Build history of the part. All positions in model axes, mm. A direction names the side the tool comes from. Give positions to 0.01 mm unless a question says otherwise; leave off trailing zeros. Order: outer loops, then holes, each group sorted by start corner. A loop starts at its lowest first (then second) coordinate and runs counter-clockwise, first axis right, second up. Notation, with made-up numbers: (48, 4) -> (104, 4) arc R24 cw to (104, 23) -> close; hole circle Ø10 at (-30.5, 24.25). An arc over 180 degrees is marked (long way). Write item = value, one per line. Start each with the question number.
from build123d import *

# Parameters (mm, degrees)
SKETCH_1_W                = 266.4
SKETCH_1_H                = 50
EXTRUDE_1_DEPTH           = 22
SKETCH_2_W                = 25.2
SKETCH_2_H                = 16
CUT_EXTRUDE_1_DEPTH       = 144.966107122
SKETCH_5_W                = 130
SKETCH_5_H                = 43
CUT_EXTRUDE_4_DEPTH       = 10
CUT_EXTRUDE_2_DEPTH       = 138.299817917
EXTRUDE_2_DEPTH           = 22
CUT_EXTRUDE_5_DEPTH       = 250
HOLE_WIZARD_1_D           = 11
HOLE_WIZARD_1_DEPTH       = 100
HOLE_WIZARD_1_CBORE_D     = 17.5
HOLE_WIZARD_1_CBORE_DEPTH = 11
SKETCH_10_R               = 10
CUT_EXTRUDE_6_DEPTH       = 2
M6X1_0_1_AT_2_COUNT       = 2
M6X1_0_1_AT_2_PITCH       = 35
FILLET_1_R                = 3


with BuildPart() as part:
    # 草图1 → 凸台-拉伸1 (new body)
    with BuildSketch(Plane.XY):
        Rectangle(SKETCH_1_W, SKETCH_1_H)
    extrude(amount=-EXTRUDE_1_DEPTH)

    # 草图2 → 切除-拉伸1 (cut, through all)
    with BuildSketch(Plane(origin=(0, 25, 0), x_dir=(1, 0, 0), z_dir=(0, 1, 0))):
        with Locations((-120.6, 14)):
            Rectangle(SKETCH_2_W, SKETCH_2_H)
        with Locations((120.6, 14)):
            Rectangle(SKETCH_2_W, SKETCH_2_H)
    extrude(amount=-CUT_EXTRUDE_1_DEPTH, mode=Mode.SUBTRACT)

    # 草图5 → 切除-拉伸4 (cut)
    with BuildSketch(Plane(origin=(0, 0, -22), x_dir=(-1, 0, 0), z_dir=(0, 0, -1))):
        with Locations((0, 3.5)):
            Rectangle(SKETCH_5_W, SKETCH_5_H)
    extrude(amount=-CUT_EXTRUDE_4_DEPTH, mode=Mode.SUBTRACT)

    # 草图3 → 切除-拉伸2 (cut, through all)
    with BuildSketch(Plane.XY):
        with BuildLine():
            Line((-42, 25), (-42, -5.726706901))
            ThreePointArc((-42, -5.726706901), (0, -18), (42, -5.726706901))
            Line((42, -5.726706901), (42, 25))
            Line((42, 25), (-42, 25))
        make_face()
    extrude(amount=-CUT_EXTRUDE_2_DEPTH, mode=Mode.SUBTRACT)

    # 草图6 → 凸台-拉伸2 (add)
    with BuildSketch(Plane.XY):
        with BuildLine():
            Line((-52.5, -25), (52.5, -25))
            ThreePointArc((52.5, -25), (0, -39.889777347), (-52.5, -25))
        make_face()
    extrude(amount=-EXTRUDE_2_DEPTH)

    # 草图7 → 切除-拉伸5 (cut, symmetric)
    with BuildSketch(Plane(origin=(0, 0, 0), x_dir=(0, 0, -1), z_dir=(1, 0, 0))):
        Polygon((22, -39.889777347), (22, -26.889777347), (9, -39.889777347), align=None)
        Polygon((0, -39.889777347), (2.7, -39.889777347), (0, -28.889777347), align=None)
    extrude(amount=CUT_EXTRUDE_5_DEPTH, both=True, mode=Mode.SUBTRACT)

    # 孔1
    with Locations(Plane.XY):
        with Locations((80, 0), (-80, 0)):
            CounterBoreHole(HOLE_WIZARD_1_D / 2, HOLE_WIZARD_1_CBORE_D / 2, HOLE_WIZARD_1_CBORE_DEPTH, depth=HOLE_WIZARD_1_DEPTH)

    # 草图10 → 切除-拉伸6 (cut)
    with BuildSketch(Plane(origin=(0, 0, -22), x_dir=(-1, 0, 0), z_dir=(0, 0, -1))):
        with Locations((80, 0)):
            Circle(SKETCH_10_R)
        with Locations((-80, 0)):
            Circle(SKETCH_10_R)
    extrude(amount=-CUT_EXTRUDE_6_DEPTH, mode=Mode.SUBTRACT)

    # 草图11 → M6x1.0 螺纹孔1 (revolve, cut)
    with BuildSketch(Plane(origin=(-108, -17.5, -13.5), x_dir=(0, 0, 1), z_dir=(0, 1, 0))):
        Polygon((0, 0), (0, 16.502151548), (2.5, 15), (2.5, 0), align=None)
    m6x1_0_1 = revolve(axis=Axis((-114.35, -17.5, -13.5), (1, 0, 0)), mode=Mode.SUBTRACT)

    # M6x1.0 螺纹孔1 at 2: M6x1.0 螺纹孔1 ×2
    with Locations(*[(0, i * M6X1_0_1_AT_2_PITCH, 0) for i in range(1, M6X1_0_1_AT_2_COUNT)]):
        add(m6x1_0_1, mode=Mode.SUBTRACT)

    # 镜向1: M6x1.0 螺纹孔1 across plane
    add(m6x1_0_1.mirror(Plane(origin=(0, 0, 0), x_dir=(0, 0, 1), z_dir=(1, 0, 0))), mode=Mode.SUBTRACT)

    # 镜向1 copy 1 sketch → 镜向1 copy 1 (revolve, cut)
    with BuildSketch(Plane(origin=(108, 17.5, -13.5), x_dir=(0, 0, 1), z_dir=(0, 1, 0))):
        Polygon((0, 0), (0, -16.502151548), (2.5, -15), (2.5, 0), align=None)
    revolve(axis=Axis((114.35, 17.5, -13.5), (1, 0, 0)), mode=Mode.SUBTRACT)

    # 圆角1
    fillet_1_edges = [part.edges().sort_by_distance(p)[0] for p in [
        (-133.2, -25, -3),
        (-133.2, 25, -3),
        (133.2, -25, -3),
        (133.2, 25, -3),
        (65, -18, -17),
        (65, 25, -17),
        (-65, 25, -17),
        (-65, -18, -17),
        (-42, 25, -6),
        (42, 25, -6),
    ]]
    fillet(fillet_1_edges, radius=FILLET_1_R)


solid = part.part
(1) Cut at C-C, the plane x = 114.5. Give the cut face in (y, z).
(2) Flat gauge pins, fed straight in: P1, Ø8, axis at y = -10, z = -12.5, coming from the +X side; P2, Ø1, axis at x = 92, y = -21, coming from the +Z side; P3, Ø6, axis at x = 29.5, z = -11.5, coming from the +Y side; P4, Ø20, axis at x = -118.5, y = -12, coming from the -Z side. Where does each tip first touch, or does it go through?
(3) Wall check: line 1 (X direction, y = 7, z = -17); line 2 (Z direction, x = 105.25, y = -17.5); line 3 (Y direction, x = 107, z = -13.25). Give the ranges that are in metal, low to high. Write a range as [from, to].
(4) 3-axis set-ups, long thin cutter, end or side, ignore diameter. For faces 1 (the face through (90, 0, -21)), 2 (the face through (-56, -1, -12)), 3 (the face through (-100.6, -19.19, -15.34)), 4 (the face through (100.6, -19.19, -15.34)): which of +Z, -Z, +X, -X, +Y, -Y reach the whole face in a straight line?
(5) Mould opens along X. For faces 5 (the face through (82, -25, -11)), 6 (the face through (-88.74, 0.38, -5.42)) say: released by +X, released by -X, zero draft, split by the parting line, or undercut.
(6) Cut at B-B, the plane y = 0. Give the number of separate pieces and of enclosed holes in the cut face, plus the area to 3 significant figures.
(7) Cut at D-D, the plane y = -31.5. Give the cut face in (x, z).
(8) Cut at A-A, the plane x = -80. Give the cut face in (y, z).
Results:
q1.outline = (-25, -6) -> (25, -6) -> (25, 0) -> (-25, 0) -> close
q2.P1 = 108
q2.P2 = 0
q2.P3 = -10.91
q2.P4 = -6
q3.line_1 = [-108, -65], [65, 108]
q3.line_2 = [-22, -16], [-11, 0]
q3.line_3 = [-25, -19.99], [-15.01, 15.01], [19.99, 25]
q4.face_1 = -Z
q4.face_2 = -Z, +Y
q4.face_3 = -X
q4.face_4 = +X
q5.face_5 = zero draft
q5.face_6 = undercut
q6.separate_pieces = 4
q6.enclosed_holes = 0
q6.area = 2,080 mm2
q7.outline = (-40.09, -17.39) -> (40.09, -17.39) -> (40.09, -0.64) -> (-40.09, -0.64) -> close
q8.outline = (-25, -22) -> (-10, -22) -> (-10, -20) -> (-5.5, -20) -> (-5.5, -11) -> (-8.75, -11) -> (-8.75, 0) -> (-25, 0) -> close; (5.5, -20) -> (10, -20) -> (10, -22) -> (25, -22) -> (25, 0) -> (8.75, 0) -> (8.75, -11) -> (5.5, -11) -> close
